```python
from build123d import *

# Parameters (mm, degrees)
SKETCH011_R     = 1.65
PAD005_DEPTH    = 3
SKETCH012_W     = 10
SKETCH012_H     = 2
POCKET007_DEPTH = 150.001
FILLET002_R     = 1.9
CHAMFER009_SIZE = 2
CHAMFER010_SIZE = 0.4


with BuildPart() as part:
    # Sketch011 (on Face1 of CopyChamfer008) → Pad005 (new body)
    with BuildSketch(Plane.XY.offset(-3.5)):
        Polygon((130, 0), (-20, 0), (-20, -12), (-3, -12), (-3, -20), (22, -20), (30, -12), (80, -12), (88, -20), (113, -20), (113, -12), (130, -12), align=None)
        with Locations((10, -16)):
            Circle(SKETCH011_R, mode=Mode.SUBTRACT)
        with Locations((100, -16)):
            Circle(SKETCH011_R, mode=Mode.SUBTRACT)
    extrude(amount=PAD005_DEPTH)

    # Sketch012 (on Face2 of Pad005) → Pocket007 (cut, through all)
    with BuildSketch(Plane(origin=(-20, 0, 0), x_dir=(0, -1, 0), z_dir=(-1, 0, 0))):
        with Locations((6, -2.5)):
            Rectangle(SKETCH012_W, SKETCH012_H)
    extrude(amount=-POCKET007_DEPTH, mode=Mode.SUBTRACT)

    # Fillet002
    fillet002_edges = [part.edges().sort_by_distance(p)[0] for p in [
        (55, -1, -1.5),
        (55, -11, -1.5),
    ]]
    fillet(fillet002_edges, radius=FILLET002_R)

    # Chamfer009
    chamfer009_edges = [part.edges().sort_by_distance(p)[0] for p in [
        (-3, -20, -2),
        (113, -20, -2),
    ]]
    chamfer(chamfer009_edges, length=CHAMFER009_SIZE)

    # Chamfer010
    chamfer010_edges = [part.edges().sort_by_distance(p)[0] for p in [
        (-3, -15, -0.5),
        (-2, -19, -0.5),
        (-11.5, -12, -0.5),
        (10.5, -20, -0.5),
        (-20, -6, -0.5),
        (26, -16, -0.5),
        (55, 0, -0.5),
        (55, -12, -0.5),
        (130, -6, -0.5),
        (84, -16, -0.5),
        (121.5, -12, -0.5),
        (99.5, -20, -0.5),
        (113, -15, -0.5),
        (112, -19, -0.5),
        (8.35, -16, -0.5),
        (98.35, -16, -0.5),
        (8.35, -16, -3.5),
        (98.35, -16, -3.5),
    ]]
    chamfer(chamfer010_edges, length=CHAMFER010_SIZE)


solid = part.part
```
Build history of the part. All positions in model axes, mm. A direction names the side the tool comes from. Round coordinates to 2 decimals unless told otherwise and drop trailing zeros. Write each loop counter-clockwise with the first axis right and the second up, starting at its lowest first coordinate (ties: lowest second). Pieces come first, ordered by that corner, then holes. Notation, with made-up numbers: (44.5, -2) - (54.5, -2) arc R31 ccw to (54.5, 30) - close; hole circle Ø5 at (4.5, 20). An arc over 180 degrees is marked (long way). Write each question's results on one line, items separated by ' | '. Start each with the question number.
Item 1: Saw through at D-D (x = 32). Write the cut outline in (y, z), and give its area (3 significant figures).
Item 2: Mould opens along Y. For faces 1 (the face through (98.35, -15.93, -2.02)), 2 (the face through (-3, -15, -2)), 3 (the face through (25.858, -15.855, -0.697)) say: pulls with the +Y half, pulls with the -Y half, needs draft (parallel to the pull), parting line crosses it, or undercut.
Item 3: Drop flat-ended pins along their axis: P1, Ø1.3, axis at y = -16, z = -2, coming from the +X side; P2, Ø0.8, axis at y = -14.5, z = -3, coming from the -X side; P3, Ø3, axis at x = 42.5, y = -7, coming from the -Z side. Give the stop position or say it passes through.
Item 4: Saw through at C-C (y = -16). Write the cut outline in (x, z).
Item 5: Which spindle directions (+Z, -Z, +X, -X, +Y, -Y) get a long thin tool onto all of the face, cutting with end or side? Do faces 4 (the face through (121, -12, -2)), 5 (the face through (84.028, -15.741, -0.697)), 6 (the face through (-12, -12, -2)). Say none if no direction does.
Item 6: Wall check: L1, parallel to X at y = -16.75, z = -1.55; L2, parallel to Y at x = 51.5, z = -3.15; L3, parallel to X at y = -15.5, z = -3.05. Give the ranges that are in metal, low to high. Write a range as [from, to].
Item 7: Saw through at B-B (x = 10). Write the cut outline in (y, z).
Item 8: Saw through at A-A (z = -2.15). Write the cut outline in (x, y), and give its area (3 significant figures).
Results are:
1) outline: (-12, -3.5) - (-11, -3.5) - (-11, -3.4) arc R1.9 cw to (-9.1, -1.5) - (-2.9, -1.5) arc R1.9 cw to (-1, -3.4) - (-1, -3.5) - (0, -3.5) - (0, -0.9) - (-0.4, -0.5) - (-11.6, -0.5) - (-12, -0.9) - close | area: 17.4 mm²
2) face 1: undercut | face 2: needs draft | face 3: pulls with the -Y half
3) P1: stops at x = 113 | P2: stops at x = -3 | P3: stops at z = -1.5
4) outline: (-3, -3.5) - (7.95, -3.5) - (8.35, -3.1) - (8.35, -0.9) - (7.95, -0.5) - (-2.6, -0.5) - (-3, -0.9) - close; (11.65, -3.1) - (12.05, -3.5) - (26, -3.5) - (26, -0.9) - (25.43, -0.5) - (12.05, -0.5) - (11.65, -0.9) - close; (84, -3.5) - (97.95, -3.5) - (98.35, -3.1) - (98.35, -0.9) - (97.95, -0.5) - (84.57, -0.5) - (84, -0.9) - close; (101.65, -3.1) - (102.05, -3.5) - (113, -3.5) - (113, -0.9) - (112.6, -0.5) - (102.05, -0.5) - (101.65, -0.9) - close
5) face 4: +Z, -Z, +X, -Y | face 5: +Z, -Y | face 6: +Z, -Z, -X, -Y
6) L1: x = [-3, 8.53], [11.47, 25.25], [84.75, 98.53], [101.47, 113] | L2: y = [-12, -10.98], [-1.02, 0] | L3: x = [-3, 8.43], [11.57, 26.5], [83.5, 98.43], [101.57, 113]
7) outline: (-20, -3.5) - (-18.05, -3.5) - (-17.65, -3.1) - (-17.65, -0.9) - (-18.05, -0.5) - (-19.6, -0.5) - (-20, -0.9) - close; (-14.35, -3.1) - (-13.95, -3.5) - (-11, -3.5) - (-11, -3.4) arc R1.9 cw to (-9.1, -1.5) - (-2.9, -1.5) arc R1.9 cw to (-1, -3.4) - (-1, -3.5) - (0, -3.5) - (0, -0.9) - (-0.4, -0.5) - (-13.95, -0.5) - (-14.35, -0.9) - close
8) outline: (-20, -12) - (-3, -12) - (-3, -18) - (-1, -20) - (22, -20) - (30, -12) - (80, -12) - (88, -20) - (111, -20) - (113, -18) - (113, -12) - (130, -12) - (130, -10.53) - (-20, -10.53) - close; (-20, -1.47) - (130, -1.47) - (130, 0) - (-20, 0) - close; hole circle Ø3.3 at (10, -16); hole circle Ø3.3 at (100, -16) | area: 884 mm²
